```python
from build123d import *

# Parameters (mm, degrees)
BRIDA_BASE1_DEPTH             = 4
PLIEGUE_START                 = -1.07192
PLIEGUE_CROQUIZADO1_OUTLINE_W = 400
PLIEGUE_CROQUIZADO1_OUTLINE_H = 4
PLIEGUE_CROQUIZADO1_DEPTH     = 33.82192
PLIEGUE_START_2               = -4.25
PLIEGUE_CROQUIZADO1_2_DEPTH   = 0.02192
PLIEGUE_START_3               = -8.25
PLIEGUE_CROQUIZADO1_3_DEPTH   = 8
PLIEGUE_START_4               = -200
PLIEGUE_CROQUIZADO1_4_DEPTH   = 400
CROQUIS8_R                    = 7
CORTAR_EXTRUIR2_DEPTH         = 10
CORTAR_EXTRUIR3_REACH         = 207.381
CROQUIS9_R                    = 2.5


with BuildPart() as part:
    # Brida base1: sheet metal written as solids
    # Croquis1 → Brida base1 (new body)
    with BuildSketch(Plane(origin=(0, 0, 0), x_dir=(1, 0, 0), z_dir=(0, 1, 0))):
        with BuildLine():
            Line((168, -32.75), (190, -32.75))
            ThreePointArc((190, -32.75), (197.071067812, -29.821067812), (200, -22.75))
            Line((200, -22.75), (200, 22.75))
            ThreePointArc((200, 22.75), (197.071067812, 29.821067812), (190, 32.75))
            Line((190, 32.75), (-190, 32.75))
            ThreePointArc((-190, 32.75), (-197.071067812, 29.821067812), (-200, 22.75))
            Line((-200, 22.75), (-200, -22.75))
            ThreePointArc((-200, -22.75), (-197.071067812, -29.821067812), (-190, -32.75))
            Line((-190, -32.75), (-168, -32.75))
            ThreePointArc((-168, -32.75), (-162.343145751, -30.406854249), (-160, -24.75))
            Line((-160, -24.75), (-160, -23.75))
            ThreePointArc((-160, -23.75), (-157.656854249, -18.093145751), (-152, -15.75))
            Line((-152, -15.75), (152, -15.75))
            ThreePointArc((152, -15.75), (157.656854249, -18.093145751), (160, -23.75))
            Line((160, -23.75), (160, -24.75))
            ThreePointArc((160, -24.75), (162.343145751, -30.406854249), (168, -32.75))
        make_face()
    extrude(amount=-BRIDA_BASE1_DEPTH)

    # Pliegue croquizado1: read off the stored shape, not the designer's step
    # Pliegue croquizado1 outline → Pliegue croquizado1 (cut)
    with BuildSketch(Plane.XY.offset(PLIEGUE_START)):
        with Locations((0, -2)):
            Rectangle(PLIEGUE_CROQUIZADO1_OUTLINE_W, PLIEGUE_CROQUIZADO1_OUTLINE_H)
    extrude(amount=PLIEGUE_CROQUIZADO1_DEPTH, mode=Mode.SUBTRACT)

    # Pliegue croquizado1 2 outline → Pliegue croquizado1 2 (add)
    with BuildSketch(Plane.XY.offset(PLIEGUE_START_2)):
        with BuildLine():
            ThreePointArc((-190, 36.999999998), (-197.071067812, 34.07106781), (-200, 26.999999998))
            Line((-200, 26.999999998), (-200, 0))
            Line((-200, 0), (200, 0))
            Line((200, 0), (200, 26.999999998))
            ThreePointArc((200, 26.999999998), (197.071067812, 34.07106781), (190, 36.999999998))
            Line((190, 36.999999998), (168, 36.999999998))
            ThreePointArc((168, 36.999999998), (162.343145751, 34.656854247), (160, 28.999999998))
            Line((160, 28.999999998), (160, 27.999999998))
            ThreePointArc((160, 27.999999998), (157.656854249, 22.343145749), (152, 19.999999998))
            Line((152, 19.999999998), (-152, 19.999999998))
            ThreePointArc((-152, 19.999999998), (-157.656854249, 22.343145749), (-160, 27.999999998))
            Line((-160, 27.999999998), (-160, 28.999999998))
            ThreePointArc((-160, 28.999999998), (-162.343145751, 34.656854248), (-168, 36.999999998))
            Line((-168, 36.999999998), (-190, 36.999999998))
        make_face()
    extrude(amount=PLIEGUE_CROQUIZADO1_2_DEPTH)

    # Pliegue croquizado1 3 outline → Pliegue croquizado1 3 (add)
    with BuildSketch(Plane.XY.offset(PLIEGUE_START_3)):
        with BuildLine():
            ThreePointArc((-190, 36.999999998), (-197.071067812, 34.07106781), (-200, 26.999999998))
            Line((-200, 26.999999998), (-200, 0))
            Line((-200, 0), (200, 0))
            Line((200, 0), (200, 26.999999998))
            ThreePointArc((200, 26.999999998), (197.071067812, 34.07106781), (190, 36.999999998))
            Line((190, 36.999999998), (168, 36.999999998))
            ThreePointArc((168, 36.999999998), (162.343145751, 34.656854247), (160, 28.999999998))
            Line((160, 28.999999998), (160, 27.999999998))
            ThreePointArc((160, 27.999999998), (157.656854249, 22.343145749), (152, 19.999999998))
            Line((152, 19.999999998), (-152, 19.999999998))
            ThreePointArc((-152, 19.999999998), (-157.656854249, 22.343145749), (-160, 27.999999998))
            Line((-160, 27.999999998), (-160, 28.999999998))
            ThreePointArc((-160, 28.999999998), (-162.343145751, 34.656854248), (-168, 36.999999998))
            Line((-168, 36.999999998), (-190, 36.999999998))
        make_face()
    extrude(amount=PLIEGUE_CROQUIZADO1_3_DEPTH)

    # Pliegue croquizado1 4 outline → Pliegue croquizado1 4 (cut)
    with BuildSketch(Plane.YZ.offset(PLIEGUE_START_4)):
        with BuildLine():
            ThreePointArc((-4, -8.25), (-1.656854249, -2.593145751), (4, -0.25))
            Line((4, -0.25), (0, -0.25))
            Line((0, -0.25), (0, -1.07192))
            Line((0, -1.07192), (-4, -1.07192))
            Line((-4, -1.07192), (-4, -8.25))
        make_face()
        with BuildLine():
            ThreePointArc((4, -4.25), (1.171572875, -5.421572875), (0, -8.25))
            Line((0, -8.25), (36.999999998, -8.25))
            Line((36.999999998, -8.25), (36.999999998, -4.25))
            Line((36.999999998, -4.25), (4, -4.25))
        make_face()
    extrude(amount=PLIEGUE_CROQUIZADO1_4_DEPTH, mode=Mode.SUBTRACT)

    # Croquis8 → Cortar-Extruir2 (cut)
    with BuildSketch(Plane(origin=(0, 0, 0), x_dir=(1, 0, 0), z_dir=(0, 1, 0))):
        with Locations(Location((0, 17.75, 0), (0, 0, 270))):
            Circle(CROQUIS8_R)
    extrude(amount=-CORTAR_EXTRUIR2_DEPTH, mode=Mode.SUBTRACT)

    # Croquis9 → Cortar-Extruir3 (cut, up to next)
    with BuildSketch(Plane(origin=(0, 0, -4.25), x_dir=(-1, 0, 0), z_dir=(0, 0, -1)), mode=Mode.PRIVATE) as cortar_extruir3_sk1:
        with Locations(Location((179, 11.999999998, 0), (0, 0, 90))):
            Circle(CROQUIS9_R)
    cortar_extruir3_tool1 = extrude(cortar_extruir3_sk1.sketch, amount=-CORTAR_EXTRUIR3_REACH, mode=Mode.PRIVATE) & part.part
    # Croquis9 → Cortar-Extruir3 (cut, up to next)
    with BuildSketch(Plane(origin=(0, 0, -4.25), x_dir=(-1, 0, 0), z_dir=(0, 0, -1)), mode=Mode.PRIVATE) as cortar_extruir3_sk2:
        with Locations(Location((179, 26.999999998, 0), (0, 0, 90))):
            Circle(CROQUIS9_R)
    cortar_extruir3_tool2 = extrude(cortar_extruir3_sk2.sketch, amount=-CORTAR_EXTRUIR3_REACH, mode=Mode.PRIVATE) & part.part
    # Croquis9 → Cortar-Extruir3 (cut, up to next)
    with BuildSketch(Plane(origin=(0, 0, -4.25), x_dir=(-1, 0, 0), z_dir=(0, 0, -1)), mode=Mode.PRIVATE) as cortar_extruir3_sk3:
        with Locations(Location((-179, 26.999999998, 0), (0, 0, 90))):
            Circle(CROQUIS9_R)
    cortar_extruir3_tool3 = extrude(cortar_extruir3_sk3.sketch, amount=-CORTAR_EXTRUIR3_REACH, mode=Mode.PRIVATE) & part.part
    # Croquis9 → Cortar-Extruir3 (cut, up to next)
    with BuildSketch(Plane(origin=(0, 0, -4.25), x_dir=(-1, 0, 0), z_dir=(0, 0, -1)), mode=Mode.PRIVATE) as cortar_extruir3_sk4:
        with Locations(Location((-179, 11.999999998, 0), (0, 0, 90))):
            Circle(CROQUIS9_R)
    cortar_extruir3_tool4 = extrude(cortar_extruir3_sk4.sketch, amount=-CORTAR_EXTRUIR3_REACH, mode=Mode.PRIVATE) & part.part
    add(cortar_extruir3_tool1.solids().sort_by_distance((-179, 12, -4.25))[0], mode=Mode.SUBTRACT)
    add(cortar_extruir3_tool2.solids().sort_by_distance((-179, 27, -4.25))[0], mode=Mode.SUBTRACT)
    add(cortar_extruir3_tool3.solids().sort_by_distance((179, 27, -4.25))[0], mode=Mode.SUBTRACT)
    add(cortar_extruir3_tool4.solids().sort_by_distance((179, 12, -4.25))[0], mode=Mode.SUBTRACT)


solid = part.part
```
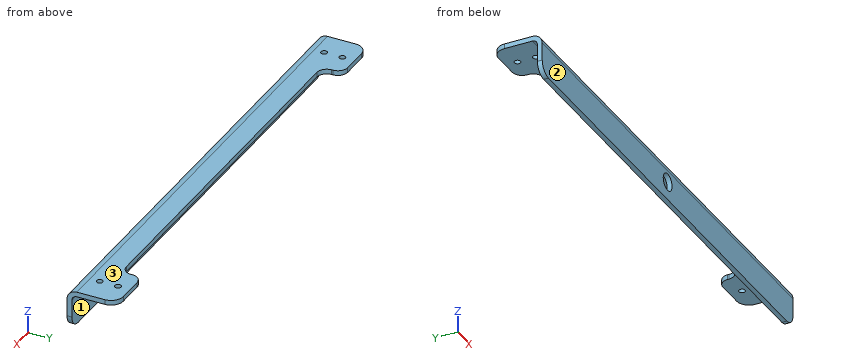
Check sheet for the modelled part. Datum: model origin and axes. Units: mm. Face numbers are marked on the shaded views. Round coordinates to 2 decimals unless told otherwise and drop trailing zeros. Order: outer loops, then holes, each group sorted by start corner. A loop starts at its lowest first (then second) coordinate and runs counter-clockwise, first axis right, second up.
1) Section check A-A (x = 0). Record the boundary of the cut face in (y, z), and give its area (3 significant figures).
2) Scan lines: line 1 (X direction, y = 12, z = -2); line 2 (X direction, y = 11.5, z = -2); line 3 (X direction, y = 27, z = -1.3). Record each from-to range of solid material in increasing order.
3) Mould release check, pull along Y, two halves, no side actions. Record for the marked faces 1, 2 and 3: +Y half, -Y half, draft (parallel to the pull), parting line (faces both ways), or undercut.
4) Section check C-C (x = 69). Record the boundary of the cut face in (y, z), and give its area (3 significant figures).
5) Section check B-B (z = -17.75). Record the boundary of the cut face in (x, y), and give its area (3 significant figures).
6) Go/stop test with flat-tipped pins: pin 1 Ø8 at (x, z) = (7, -29) entering from +Y; pin 2 Ø2 at (x, y) = (-18, 3) entering from -Z; pin 3 Ø0.8 at (y, z) = (28.5, -1.5) entering from -X. Record where each tip stops, or that it passes through.
Result:
1. outline: (-4, -32.75) - (0, -32.75) - (0, -24.75) - (-4, -24.75) - close; (-4, -10.75) - (0, -10.75) - (0, -8.25) arc R4 cw to (4, -4.25) - (20, -4.25) - (20, -0.25) - (4, -0.25) arc R8 ccw to (-4, -8.25) - close
1. area: 144 mm2
2. line 1: x = -200 to -181.5, -176.5 to 176.5, 181.5 to 200
2. line 2: x = -200 to -181.45, -176.55 to 176.55, 181.45 to 200
2. line 3: x = -200 to -181.5, -176.5 to -159.94, 159.94 to 176.5, 181.5 to 200
3. face 1: +Y half
3. face 2: -Y half
3. face 3: draft
4. outline: (-4, -32.75) - (0, -32.75) - (0, -8.25) arc R4 cw to (4, -4.25) - (20, -4.25) - (20, -0.25) - (4, -0.25) arc R8 ccw to (-4, -8.25) - close
4. area: 200 mm2
5. outline: (-200, -4) - (-7, -4) - (-7, 0) - (-200, 0) - close; (7, -4) - (200, -4) - (200, 0) - (7, 0) - close
5. area: 1,540 mm2
6. pin 1: stops at y = 0
6. pin 2: stops at z = -4.79
6. pin 3: stops at x = -199.94
